from build123d import *
from build123d.topology import SkipClean

# Parameters (mm, degrees)
SKETCH1_W               = 48
SKETCH1_H               = 53
BOSS_EXTRUDE1_DEPTH     = 10
SKETCH2_W               = 48
SKETCH2_H               = 5.616325
BOSS_EXTRUDE2_DEPTH     = 33.1917878
SKETCH4_W               = 4
SKETCH4_H               = 10
BOSS_EXTRUDE4_DEPTH     = 40
SKETCH5_W               = 48
SKETCH5_H               = 10.8609375
BOSS_EXTRUDE5_DEPTH     = 23.1917878
SKETCH6_W               = 48
SKETCH6_H               = 5
BOSS_EXTRUDE6_DEPTH     = 42.3
SKETCH7_W               = 12.8082122
SKETCH7_H               = 16.4772625
BOSS_EXTRUDE7_DEPTH     = 48
CUT_EXTRUDE1_REACH      = 84.426
SKETCH8_R               = 11.5
SKETCH8_R_2             = 2
FILLET1_R               = 10
FILLET2_R               = 4
SKETCH9_W               = 5
SKETCH9_H               = 16.4772625
BOSS_EXTRUDE9_DEPTH     = 48
CUT_EXTRUDE2_DEPTH      = 88.252507127
SKETCH11_W              = 51
SKETCH11_H              = 16.4772625
BOSS_EXTRUDE10_DEPTH    = 49.45
BOSS_EXTRUDE11_DEPTH    = 46
SKETCH16_W              = 47.95
SKETCH16_H              = 51
BOSS_EXTRUDE14_DEPTH    = 2.55
SKETCH14_W              = 5
SKETCH14_H              = 42.3
BOSS_EXTRUDE13_DEPTH    = 1.5
SKETCH17_W              = 51
SKETCH17_H              = 19.0272625
BOSS_EXTRUDE15_DEPTH    = 9
BOSS_EXTRUDE16_DEPTH    = 25
SKETCH19_R              = 1.9304
CUT_EXTRUDE3_DEPTH      = 125.404890183
MIRROR2_START           = 33.1917878
MIRROR2_DEPTH           = 51
MIRROR2_START_2         = 76.1917878
MIRROR2_2_OUTLINE_W     = 47.95
MIRROR2_2_OUTLINE_H     = 25
MIRROR2_2_OUTLINE_R     = 1.9304
MIRROR2_2_DEPTH         = 8
MIRROR2_3_OUTLINE_W     = 45
MIRROR2_3_OUTLINE_H     = 42.3
MIRROR2_3_OUTLINE_R     = 2
MIRROR2_3_OUTLINE_R_2   = 11.5
MIRROR2_3_DEPTH         = 5
SKETCH20_W              = 103.287975037
SKETCH20_H              = 97.84889924
CUT_EXTRUDE4_DEPTH      = 144.929961559
SKETCH21_W              = 49.5
SKETCH21_H              = 42.3
CUT_EXTRUDE5_DEPTH      = 128.391431036
SKETCH24_R              = 7.5
BOSS_EXTRUDE18_DEPTH    = 45
BOSS_EXTRUDE19_DEPTH    = 29
SKETCH26_R              = 3.937
CUT_EXTRUDE6_DEPTH      = 135.023808387
CUT_EXTRUDE7_DEPTH      = 133.174975247
CUT_EXTRUDE7_DEPTH_BACK = 133.174975247
SKETCH27_W              = 131.04651434
SKETCH27_H              = 69.942394415
SKETCH30_W              = 22
SKETCH30_H              = 11.4772625
SKETCH30_W_2            = 5
CUT_EXTRUDE10_DEPTH     = 95.954850856


# Read off the part's stored shape, not the designer's step: Mirror2
with BuildPart() as part:
    # Sketch1 → Boss-Extrude1 (new body)
    with BuildSketch(Plane.XY):
        with Locations((24, 26.5)):
            Rectangle(SKETCH1_W, SKETCH1_H)
    extrude(amount=BOSS_EXTRUDE1_DEPTH)

    # Sketch2 → Boss-Extrude2 (add)
    with BuildSketch(Plane(origin=(0, 0, 0), x_dir=(-1, 0, 0), z_dir=(0, 0, -1))):
        with Locations((-24, -2.8081625)):
            Rectangle(SKETCH2_W, SKETCH2_H)
    extrude(amount=-BOSS_EXTRUDE2_DEPTH)

    # Sketch4 → Boss-Extrude4 (add)
    with BuildSketch(Plane.XY.offset(10)):
        with Locations((2, 48)):
            Rectangle(SKETCH4_W, SKETCH4_H)
        with Locations((46, 48)):
            Rectangle(SKETCH4_W, SKETCH4_H)
    extrude(amount=BOSS_EXTRUDE4_DEPTH)

    # Sketch5 → Boss-Extrude5 (add)
    with BuildSketch(Plane.XY.offset(10)):
        with Locations((24, 5.43046875)):
            Rectangle(SKETCH5_W, SKETCH5_H)
    extrude(amount=BOSS_EXTRUDE5_DEPTH)

    # Sketch6 → Boss-Extrude6 (add)
    with BuildSketch(Plane.XZ.offset(5.616325)):
        with Locations((24, 30.6917878)):
            Rectangle(SKETCH6_W, SKETCH6_H)
    extrude(amount=BOSS_EXTRUDE6_DEPTH)

    # Sketch7 → Boss-Extrude7 (add)
    with BuildSketch(Plane.ZY):
        with Locations((-6.4041061, 2.62230625)):
            Rectangle(SKETCH7_W, SKETCH7_H)
    extrude(amount=-BOSS_EXTRUDE7_DEPTH)

    # Sketch8 → Cut-Extrude1 (cut, up to next)
    with BuildSketch(Plane(origin=(0, 0, 28.1917878), x_dir=(-1, 0, 0), z_dir=(0, 0, -1)), mode=Mode.PRIVATE) as cut_extrude1_sk1:
        with Locations((-24, -26.616325)):
            Circle(SKETCH8_R)
    cut_extrude1_tool1 = extrude(cut_extrude1_sk1.sketch, amount=-CUT_EXTRUDE1_REACH, mode=Mode.PRIVATE) & part.part
    # Sketch8 → Cut-Extrude1 (cut, up to next)
    with BuildSketch(Plane(origin=(0, 0, 28.1917878), x_dir=(-1, 0, 0), z_dir=(0, 0, -1)), mode=Mode.PRIVATE) as cut_extrude1_sk2:
        with Locations((-39.5, -11.116325)):
            Circle(SKETCH8_R_2)
    cut_extrude1_tool2 = extrude(cut_extrude1_sk2.sketch, amount=-CUT_EXTRUDE1_REACH, mode=Mode.PRIVATE) & part.part
    # Sketch8 → Cut-Extrude1 (cut, up to next)
    with BuildSketch(Plane(origin=(0, 0, 28.1917878), x_dir=(-1, 0, 0), z_dir=(0, 0, -1)), mode=Mode.PRIVATE) as cut_extrude1_sk3:
        with Locations((-39.5, -42.116325)):
            Circle(SKETCH8_R_2)
    cut_extrude1_tool3 = extrude(cut_extrude1_sk3.sketch, amount=-CUT_EXTRUDE1_REACH, mode=Mode.PRIVATE) & part.part
    # Sketch8 → Cut-Extrude1 (cut, up to next)
    with BuildSketch(Plane(origin=(0, 0, 28.1917878), x_dir=(-1, 0, 0), z_dir=(0, 0, -1)), mode=Mode.PRIVATE) as cut_extrude1_sk4:
        with Locations((-8.5, -11.116325)):
            Circle(SKETCH8_R_2)
    cut_extrude1_tool4 = extrude(cut_extrude1_sk4.sketch, amount=-CUT_EXTRUDE1_REACH, mode=Mode.PRIVATE) & part.part
    # Sketch8 → Cut-Extrude1 (cut, up to next)
    with BuildSketch(Plane(origin=(0, 0, 28.1917878), x_dir=(-1, 0, 0), z_dir=(0, 0, -1)), mode=Mode.PRIVATE) as cut_extrude1_sk5:
        with Locations((-8.5, -42.116325)):
            Circle(SKETCH8_R_2)
    cut_extrude1_tool5 = extrude(cut_extrude1_sk5.sketch, amount=-CUT_EXTRUDE1_REACH, mode=Mode.PRIVATE) & part.part
    add(cut_extrude1_tool1.solids().sort_by_distance((24, -26.616325, 28.191788))[0], mode=Mode.SUBTRACT)
    add(cut_extrude1_tool2.solids().sort_by_distance((39.5, -11.116325, 28.191788))[0], mode=Mode.SUBTRACT)
    add(cut_extrude1_tool3.solids().sort_by_distance((39.5, -42.116325, 28.191788))[0], mode=Mode.SUBTRACT)
    add(cut_extrude1_tool4.solids().sort_by_distance((8.5, -11.116325, 28.191788))[0], mode=Mode.SUBTRACT)
    add(cut_extrude1_tool5.solids().sort_by_distance((8.5, -42.116325, 28.191788))[0], mode=Mode.SUBTRACT)

    # Fillet1
    fillet1_edges = [part.edges().sort_by_distance(p)[0] for p in [
        (24, 10.8609375, 0),
    ]]
    fillet(fillet1_edges, radius=FILLET1_R)

    # Fillet2
    fillet2_edges = [part.edges().sort_by_distance(p)[0] for p in [
        (2, 43, 10),
        (46, 43, 10),
    ]]
    fillet(fillet2_edges, radius=FILLET2_R)

    # Sketch9 → Boss-Extrude9 (add)
    with BuildSketch(Plane(origin=(48, 0, 0), x_dir=(0, 0, -1), z_dir=(1, 0, 0))):
        with Locations((15.3082122, 2.62230625)):
            Rectangle(SKETCH9_W, SKETCH9_H)
    extrude(amount=-BOSS_EXTRUDE9_DEPTH)

    # Sketch10 → Cut-Extrude2 (cut, through all)
    with BuildSketch(Plane(origin=(48, 0, 0), x_dir=(0, 0, -1), z_dir=(1, 0, 0))):
        Polygon((17.8082122, 10.8609375), (-33.1917878, 10.8609375), (-76.887145623, 43.902095521), (-50.794096938, 74.436514195), (27.207463492, 71.105486703), align=None)
    extrude(amount=-CUT_EXTRUDE2_DEPTH, mode=Mode.SUBTRACT)

    # Sketch11 → Boss-Extrude10 (add)
    with BuildSketch(Plane(origin=(48, 0, 0), x_dir=(0, 0, -1), z_dir=(1, 0, 0))):
        with Locations((-7.6917878, 2.62230625)):
            Rectangle(SKETCH11_W, SKETCH11_H)
    extrude(amount=BOSS_EXTRUDE10_DEPTH)

    # Sketch12 → Boss-Extrude11 (add)
    with BuildSketch(Plane(origin=(0, 0, 28.1917878), x_dir=(-1, 0, 0), z_dir=(0, 0, -1))):
        Polygon((-48, -47.916325), (-45, -47.916325), (-45, -5.616325), (-49.5, -5.616325), (-49.5, -47.916325), align=None)
    extrude(amount=BOSS_EXTRUDE11_DEPTH)

    # Sketch16 → Boss-Extrude14 (add)
    with BuildSketch(Plane.XZ.offset(5.616325)):
        with Locations((73.475, 7.6917878)):
            Rectangle(SKETCH16_W, SKETCH16_H)
    extrude(amount=BOSS_EXTRUDE14_DEPTH)

    # Sketch14 → Boss-Extrude13 (add)
    with BuildSketch(Plane(origin=(49.5, 0, 0), x_dir=(0, 0, -1), z_dir=(1, 0, 0))):
        with Locations((-30.6917878, -26.766325)):
            Rectangle(SKETCH14_W, SKETCH14_H)
    extrude(amount=-BOSS_EXTRUDE13_DEPTH)

    # Sketch17 → Boss-Extrude15 (add)
    with BuildSketch(Plane(origin=(97.45, 0, 0), x_dir=(0, 0, -1), z_dir=(1, 0, 0))):
        with Locations((-7.6917878, 1.34730625)):
            Rectangle(SKETCH17_W, SKETCH17_H)
    extrude(amount=BOSS_EXTRUDE15_DEPTH)

    # Sketch18 → Boss-Extrude16 (add)
    with BuildSketch(Plane.XZ.offset(8.166325)):
        Polygon((49.5, -17.8082122), (106.45, -17.8082122), (106.45, -9.8082122), (106.45, 33.1917878), (97.45, 33.1917878), (97.45, -9.8082122), (49.5, -9.8082122), align=None)
    extrude(amount=BOSS_EXTRUDE16_DEPTH)

    # Sketch19 → Cut-Extrude3 (cut, through all)
    with BuildSketch(Plane.XY.offset(-9.8082122)):
        with Locations((58.475, -26.166325)):
            Circle(SKETCH19_R)
        with Locations((88.475, -26.166325)):
            Circle(SKETCH19_R)
    extrude(amount=-CUT_EXTRUDE3_DEPTH, mode=Mode.SUBTRACT)

    # Mirror2 outline → Mirror2 (add)
    with BuildSketch(Plane.XY.offset(MIRROR2_START)):
        Polygon((49.5, -47.916325), (49.5, -8.166325), (97.45, -8.166325), (97.45, -33.166325), (106.45, -33.166325), (106.45, 10.8609375), (0, 10.8609375), (0, -5.616325), (45, -5.616325), (45, -47.916325), align=None)
    extrude(amount=MIRROR2_DEPTH)

    # Mirror2 2 outline → Mirror2 2 (add)
    with BuildSketch(Plane.XY.offset(MIRROR2_START_2)):
        with Locations((73.475, -20.666325)):
            Rectangle(MIRROR2_2_OUTLINE_W, MIRROR2_2_OUTLINE_H)
        with Locations((58.475, -26.166325)):
            Circle(MIRROR2_2_OUTLINE_R, mode=Mode.SUBTRACT)
        with Locations((88.475, -26.166325)):
            Circle(MIRROR2_2_OUTLINE_R, mode=Mode.SUBTRACT)
    extrude(amount=MIRROR2_2_DEPTH)

    # Mirror2 3 outline → Mirror2 3 (add)
    with SkipClean():  # the faces are left unmerged after this step: merging them gives an invalid solid
        with BuildSketch(Plane.XY.offset(MIRROR2_START)):
            with Locations((22.5, -26.766325)):
                Rectangle(MIRROR2_3_OUTLINE_W, MIRROR2_3_OUTLINE_H)
            with Locations((8.5, -42.116325)):
                Circle(MIRROR2_3_OUTLINE_R, mode=Mode.SUBTRACT)
            with Locations((39.5, -42.116325)):
                Circle(MIRROR2_3_OUTLINE_R, mode=Mode.SUBTRACT)
            with Locations((24, -26.616325)):
                Circle(MIRROR2_3_OUTLINE_R_2, mode=Mode.SUBTRACT)
            with Locations((8.5, -11.116325)):
                Circle(MIRROR2_3_OUTLINE_R, mode=Mode.SUBTRACT)
            with Locations((39.5, -11.116325)):
                Circle(MIRROR2_3_OUTLINE_R, mode=Mode.SUBTRACT)
        extrude(amount=MIRROR2_3_DEPTH)

    # Sketch20 → Cut-Extrude4 (cut, through all)
    with BuildSketch(Plane.ZY):
        with Locations((-18.452199719, -38.06351212)):
            Rectangle(SKETCH20_W, SKETCH20_H)
    extrude(amount=-CUT_EXTRUDE4_DEPTH, mode=Mode.SUBTRACT)

    # Sketch21 → Cut-Extrude5 (cut, through all)
    with BuildSketch(Plane.XY.offset(84.1917878)):
        with Locations((24.75, -26.766325)):
            Rectangle(SKETCH21_W, SKETCH21_H)
    extrude(amount=-CUT_EXTRUDE5_DEPTH, mode=Mode.SUBTRACT)



with BuildPart() as body_2:
    # Sketch24 → Boss-Extrude18 (new body)
    with BuildSketch(Plane.XY.offset(55.1917878)):
        with Locations((24, -29.616325)):
            Circle(SKETCH24_R)
    extrude(amount=-BOSS_EXTRUDE18_DEPTH)


with BuildPart() as part_1:
    add(part.part)

    add(body_2.part)  # Boss-Extrude19 merges body 2
    # Sketch25 → Boss-Extrude19 (add)
    with BuildSketch(Plane.XY.offset(55.1917878)):
        with BuildLine():
            Line((16.5, -29.616325), (12.268152463, -5.616325))
            Line((12.268152463, -5.616325), (35.731847537, -5.616325))
            Line((35.731847537, -5.616325), (31.5, -29.616325))
            ThreePointArc((31.5, -29.616325), (24, -37.116325), (16.5, -29.616325))
        make_face()
    extrude(amount=BOSS_EXTRUDE19_DEPTH)

    # Sketch26 → Cut-Extrude6 (cut, through all)
    with BuildSketch(Plane.ZY.offset(-97.45)):
        with Locations((59.1917878, -16.166325)):
            Circle(SKETCH26_R)
    extrude(amount=-CUT_EXTRUDE6_DEPTH, mode=Mode.SUBTRACT)

    # Sketch27 → Cut-Extrude7 (cut, two sides: drawn at the far end of the back side and taken through both)
    with BuildSketch(Plane.XY.offset(79.1917878).offset(-CUT_EXTRUDE7_DEPTH_BACK)):
        with Locations((52.297526751, -17.773339354)):
            Rectangle(SKETCH27_W, SKETCH27_H)
        Polygon((12.268152463, -5.616325), (12.268152463, 5.8609375), (35.731847537, 5.8609375), (35.731847537, -5.616325), (35.731847537, -46.734959709), (12.268152463, -46.734959709), align=None, mode=Mode.SUBTRACT)
    extrude(amount=CUT_EXTRUDE7_DEPTH + CUT_EXTRUDE7_DEPTH_BACK, mode=Mode.SUBTRACT)

    # Sketch30 → Cut-Extrude10 (cut, through all)
    with BuildSketch(Plane.ZY.offset(-12.268152463)):
        with Locations((44.1917878, 0.12230625)):
            Rectangle(SKETCH30_W, SKETCH30_H)
        with Locations((81.6917878, 0.12230625)):
            Rectangle(SKETCH30_W_2, SKETCH30_H)
    extrude(amount=-CUT_EXTRUDE10_DEPTH, mode=Mode.SUBTRACT)


solid = part_1.part
The listing builds one solid part. Answer for the finished solid, in the listing's coordinates (mm). A direction names the side the tool comes from. Give positions to 0.01 mm unless a question says otherwise; leave off trailing zeros. Write each loop counter-clockwise with the first axis right and the second up, starting at its lowest first coordinate (ties: lowest second). Pieces come first, ordered by that corner, then holes. Notation, with made-up numbers: (59, -19.75) -> (89, -19.75) arc R22 cw to (89, -13.75) -> close; hole circle Ø2 at (-14.75, 8.5). An arc over 180 degrees is marked (long way). Use a Markdown table: item, result.
(1) Flat-ended cylindrical pins translate along their axes: P1, Ø1.5, axis at x = 32, y = -30, coming from the +Z side; P2, Ø2, axis at y = -22, z = 69.5, coming from the +X side; P3, Ø6, axis at y = -21, z = 65.5, coming from the +X side; P4, Ø5, axis at x = 29.5, z = 34, coming from the -Y side. Find the tip coordinate at first contact, or state that the pin passes through.
Return value:
| item | result |
|---|---|
| P1 | z = 84.19 |
| P2 | x = 33.02 |
| P3 | x = 33.55 |
| P4 | y = -36.49 |
(2) Section A-A, the plane z = 56 is taken. Determine the outline of the cut face in (x, y).
Return value:
| item | result |
|---|---|
| outline | (12.27, -5.62) -> (16.5, -29.62) arc R7.5 ccw to (31.5, -29.62) -> (35.73, -5.62) -> (35.73, 5.86) -> (12.27, 5.86) -> close |
(3) Find the intervals of material crossed by probe 1 along Z at (x, y) = (25.5, -4.5); probe 2 along Z at (x, y) = (23.25, -7.5); probe 3 along Y at (x, z) = (22.25, 21), in increasing order. Write a range as from..to.
Return value:
| item | result |
|---|---|
| probe 1 | 55.19..79.19 |
| probe 2 | 55.19..84.19 |
| probe 3 | -36.91..-22.32 |
(4) For faces 4 (the flat face through (24, -18, 84.192)), 5 (the flat face through (24, -5.616, 82)), 6 (the cylindrical face through (23.024, -37.053, 38.452)), determine the directions among +Z, -Z, +X, -X, +Y, -Y from which every point of the face is accessible in a straight line to the end or side of a thin tool.
Return value:
| item | result |
|---|---|
| face 4 | +Z, +X, -X, +Y, -Y |
| face 5 | +Z, +X, -X, +Y |
| face 6 | -Z |
(5) Section C-C, the plane x = 24 is taken. Determine the outline of the cut face in (y, z), then the cut area to 3 significant figures.
Return value:
| item | result |
|---|---|
| outline | (-37.12, 10.19) -> (-22.12, 10.19) -> (-22.12, 55.19) -> (5.86, 55.19) -> (5.86, 79.19) -> (-5.62, 79.19) -> (-5.62, 84.19) -> (-37.12, 84.19) -> close |
| area | 1,860 mm2 |
(6) Determine the mould class of faces 1 (the flat face through (33.646, -17.448, 69.489)), 2 (the flat face through (24, 0, 79.192)), 3 (the flat face through (24, 5.861, 67)) for opening direction Y: released by +Y, released by -Y, zero draft, split by the parting line, or undercut.
Return value:
| item | result |
|---|---|
| face 1 | released by -Y |
| face 2 | zero draft |
| face 3 | released by +Y |
(7) Section D-D, the plane x = 15 is taken. Determine the outline of the cut face in (y, z), then the cut area to 3 significant figures.
Return value:
| item | result |
|---|---|
| outline | (-21.11, 55.19) -> (5.86, 55.19) -> (5.86, 79.19) -> (-5.62, 79.19) -> (-5.62, 84.19) -> (-21.11, 84.19) -> close |
| area | 725 mm2 |
(8) Section B-B, the plane y = -28 is taken. Determine the outline of the cut face in (x, z) (3 decimals).
Return value:
| item | result |
|---|---|
| outline | (16.215, 55.192) -> (16.676, 55.192) -> (16.676, 10.192) -> (31.324, 10.192) -> (31.324, 55.192) -> (31.785, 55.192) -> (31.785, 84.192) -> (16.215, 84.192) -> close |
